Design review of the part shown in the three views and the two pictorial views. Dimensions are in mm from the part's minimum x, y and z. A direction names the side the tool comes from. Coordinates: 2 decimals unless noted, no trailing zeros. Write each loop counter-clockwise with the first axis right and the second up, starting at its lowest first coordinate (ties: lowest second). Pieces come first, ordered by that corner, then holes. Notation, with made-up numbers: M 32.5,38 L 40.5,38 A10 cw 40.5,56 Z; hole C 42,25.25 d10. An arc over 180 degrees is marked long. Answer as a JSON object with one key per item and string values.
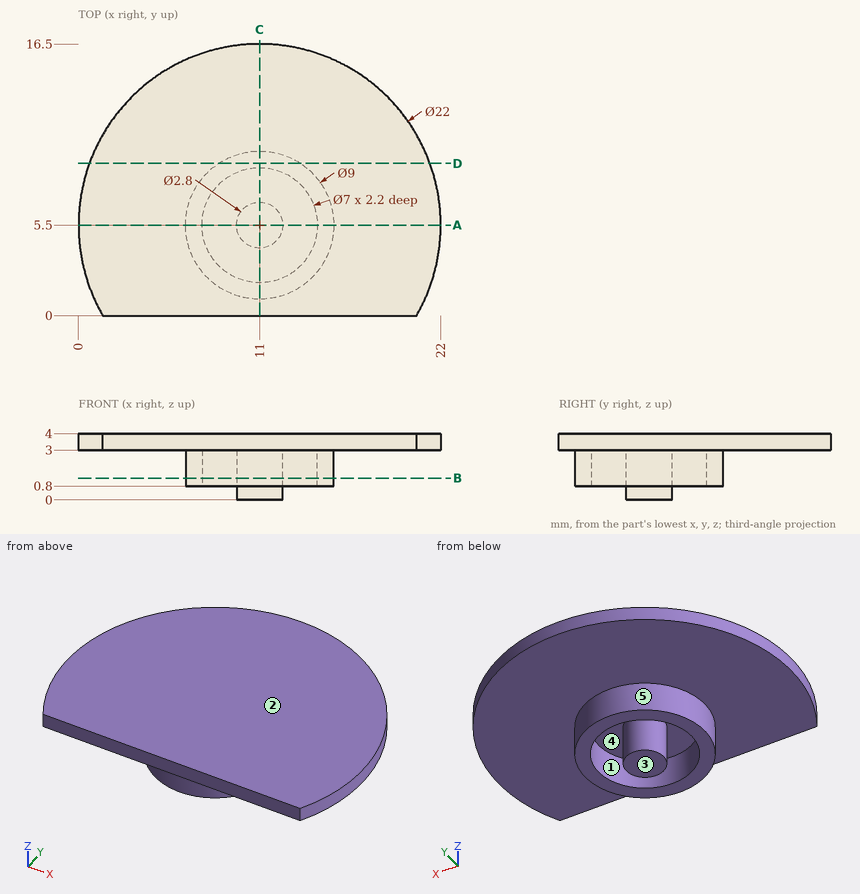
(1) Add section B-B on z = 1.3. Give the boundary of the cut face in (x, y), and give its area (3 significant figures).
Results list:
{"outline": "C 11,5.5 d9; C 11,5.5 d2.8; hole C 11,5.5 d7", "area": "31.3 mm²"}
(2) For pin 1 Ø7 at (x, y) = (9.5, 3.5) entering from -Z; pin 2 Ø5 at (x, y) = (11.5, 10) entering from -Z; pin 3 Ø1 at (x, y) = (19.5, 12) entering from -Z; pin 4 Ø2 at (y, z) = (9.5, 3) entering from +X, all flat-tipped, find the tip position at first contact; note any pin that passes through.
Results list:
{"pin 1": "z = 0", "pin 2": "z = 0.8", "pin 3": "z = 3", "pin 4": "x = 21.58"}
(3) For the marked faces 1 and 2, list the 3-axis set-ups (+Z, -Z, +X, -X, +Y, -Y) from which the entire face can be reached by the end or side of a thin tool; tool diameter is ignored.
Results list:
{"face 1": "-Z", "face 2": "+Z, +X, -X, +Y, -Y"}
(4) Wall thickness on line 1 along Y through (x, z) = (11, 2.35); line 2 along Z through (x, y) = (18, 8.75); line 3 along Z through (x, y) = (10.5, 9.75): over which ranges is each line inside the solid? List them lowest first. Write a range as from..to.
Results list:
{"line 1": "1..2, 4.1..6.9, 9..10", "line 2": "3..4", "line 3": "0.8..4"}
(5) Add section A-A on y = 5.5. Give the boundary of the cut face in (x, z), and give its area (3 significant figures).
Results list:
{"outline": "M 0,3 L 6.5,3 L 6.5,0.8 L 7.5,0.8 L 7.5,3 L 9.6,3 L 9.6,0 L 12.4,0 L 12.4,3 L 14.5,3 L 14.5,0.8 L 15.5,0.8 L 15.5,3 L 22,3 L 22,4 L 0,4 Z", "area": "34.8 mm²"}
(6) Draft analysis for pull direction Y (two halves, no side actions). For the marked faces 3, 4 and 5, state which applies: released by +Y, released by -Y, zero draft, split by the parting line, or undercut.
Results list:
{"face 3": "zero draft", "face 4": "undercut", "face 5": "split by the parting line"}
(7) Add section D-D on y = 9.25. Give the boundary of the cut face in (x, z), and give its area (3 significant figures).
Results list:
{"outline": "M 0.66,3 L 8.51,3 L 8.51,0.8 L 13.49,0.8 L 13.49,3 L 21.34,3 L 21.34,4 L 0.66,4 Z", "area": "31.6 mm²"}
(8) Add section C-C on x = 11. Give the boundary of the cut face in (y, z).
Results list:
{"outline": "M 0,3 L 1,3 L 1,0.8 L 2,0.8 L 2,3 L 4.1,3 L 4.1,0 L 6.9,0 L 6.9,3 L 9,3 L 9,0.8 L 10,0.8 L 10,3 L 16.5,3 L 16.5,4 L 0,4 Z"}
